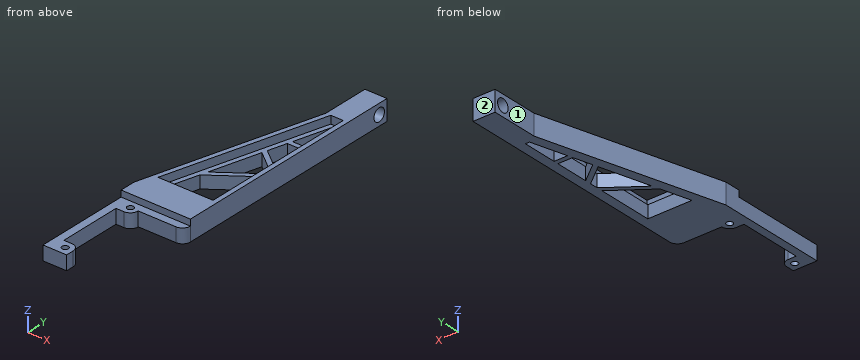
```python
from build123d import *

# Parameters (mm, degrees)
F1_DEPTH  = 13
F0_R      = 2
F2_DEPTH  = 9
F4_DEPTH  = 5
F6_DEPTH  = 8.001
F7_R      = 5
F8_R      = 4.99999
F9_R      = 5
F10_R     = 4.05
F11_DEPTH = 14.001


# Not quite as in the source:
# - a fillet or chamfer is up to 0.001 mm smaller than in the source, because OpenCascade refuses the exact size


with BuildPart() as f1:
    # F0 (on Top) → F1 (new body)
    with BuildSketch(Plane.XY):
        Polygon((-22.5616768954, -33.6060966955), (21.4383231046, -33.6060966955), (21.4383231046, 117.3939033045), (7.4383231046, 117.3939033045), (7.4383231046, 87.3939033045), (-22.5616768954, -23.6060966955), align=None)
    extrude(amount=F1_DEPTH)

    # F0 (on Top) → F2 (join)
    with BuildSketch(Plane.XY):
        Polygon((-17.5616768954, -43.6060966955), (-7.5616768954, -43.6060966955), (-7.5616768954, -38.6060966955), (21.4383231046, -38.6060966955), (21.4383231046, -33.6060966955), (-22.5616768954, -33.6060966955), (-22.5616768954, -93.6060966955), (-7.5616768954, -93.6060966955), (-7.5616768954, -83.6060966955), (-17.5616768954, -83.6060966955), align=None)
        with Locations((-12.5616768954, -88.6060966955)):
            Circle(F0_R, mode=Mode.SUBTRACT)
        with Locations((-12.5616768954, -38.6060966955)):
            Circle(F0_R, mode=Mode.SUBTRACT)
    extrude(amount=F2_DEPTH)

    # F3 (on face) → F4 (cut)
    with BuildSketch(Plane.XY.offset(13)):
        Polygon((-16.4810658851, -12.6060966955), (18.4383231046, -12.6060966955), (18.4383231046, 87.3939033045), (10.545961142, 87.3939033045), align=None)
    extrude(amount=-F4_DEPTH, mode=Mode.SUBTRACT)

    # F5 (on face) → F6 (cut, through all)
    with BuildSketch(Plane.XY.offset(8)):
        Polygon((15.4383231046, 62.3939033045), (15.4383231046, 84.3939033045), (12.8427883685, 84.3939033045), (6.8968424225, 62.3939033045), align=None)
        Polygon((15.4383231046, 38.1328739976), (15.4383231046, 59.3939033045), (6.0860316117, 59.3939033045), (2.95512331, 47.8095425882), align=None)
        Polygon((15.4383231046, 29.3370774792), (15.4383231046, 34.3370774792), (2.1069338573, 44.6712416135), (-6.3520655178, 13.3729439254), align=None)
        Polygon((15.4383231046, -9.6060966955), (15.4383231046, 25.6181227456), (-7.6053455592, 8.7358077721), (-12.562617037, -9.6060966955), align=None)
    extrude(amount=-F6_DEPTH, mode=Mode.SUBTRACT)

    # F7
    f7_edges = [f1.edges().sort_by_distance(p)[0] for p in [
        (21.438323, -38.606097, 4.5),
    ]]
    fillet(f7_edges, radius=F7_R)

    # F8 (radius 5 in the source; OpenCascade refuses exactly that, so slightly less here)
    f8_edges = [f1.edges().sort_by_distance(p)[0] for p in [
        (-7.561677, -43.606097, 4.5),
    ]]
    fillet(f8_edges, radius=F8_R)

    # F9
    f9_edges = [f1.edges().sort_by_distance(p)[0] for p in [
        (-7.561677, -83.606097, 4.5),
    ]]
    fillet(f9_edges, radius=F9_R)

    # F10 (on face) → F11 (cut, through all)
    with BuildSketch(Plane(origin=(7.4383231046, 0, 0), x_dir=(0, -1, 0), z_dir=(-1, 0, 0))):
        with Locations((-111.3939033045, 6.5)):
            Circle(F10_R)
    extrude(amount=-F11_DEPTH, mode=Mode.SUBTRACT)


solid = f1.part
```
Part model, mm, in its own coordinate system. Face numbers are marked on the shaded views. A direction names the side the tool comes from. Round coordinates to 2 decimals unless told otherwise and drop trailing zeros. Loops run counter-clockwise (first coordinate to the right, second up) from the corner with the lowest first, then second, coordinate; pieces in that order, holes last.
Item 1: Cut at A-A, the plane x = -0.5. Give the cut face in (y, z), then the cut area to 3 significant figures.
Item 2: 3-axis set-ups, long thin cutter, end or side, ignore diameter. For the marked faces 1 and 2: which of +Z, -Z, +X, -X, +Y, -Y reach the whole face in a straight line?
Item 3: Drill centre lines: line 1 (X direction, y = 97.5, z = 11.25); line 2 (X direction, y = 12, z = 11.5); line 3 (Z direction, x = 5, y = 65.5). Where is each one in solid material? Low to high.
Item 4: Drop flat-ended pins along their axis: P1, Ø1, axis at x = -11.5, y = -18.5, coming from the -Z side; P2, Ø2.5, axis at y = 42.5, z = 11.5, coming from the -X side; P3, Ø5, axis at y = -12.5, z = 1.5, coming from the -X side; P4, Ø4, axis at y = 31.5, z = 5, coming from the -X side. Give the stop position or say it passes through.
Item 5: Cut at B-B, the plane y = 97.5. Give the cut face in (x, z).
A:
1. outline: (-38.61, 0) - (-9.61, 0) - (-9.61, 8) - (-12.61, 8) - (-12.61, 13) - (-33.61, 13) - (-33.61, 9) - (-38.61, 9) - close; (13.94, 0) - (17.66, 0) - (17.66, 8) - (13.94, 8) - close; (35.03, 0) - (58.02, 0) - (58.02, 13) - (46.52, 13) - (46.52, 8) - (35.03, 8) - close
1. area: 613 mm2
2. face 1: +Z, -Z, -X, +Y
2. face 2: +Z, -Z, +X, -X, +Y
3. line 1: x = 7.44 to 21.44
3. line 2: x = -12.94 to -9.83, 18.44 to 21.44
3. line 3: z = 0 to 8
4. P1: stops at z = 0
4. P2: stops at x = -5.03
4. P3: stops at x = -20.24
4. P4: stops at x = -8.21
5. outline: (7.44, 0) - (21.44, 0) - (21.44, 13) - (7.44, 13) - close
